```python
from build123d import *

# Parameters (mm, degrees)
SKETCH1_W                   = 88.6
SKETCH1_H                   = 35
BOSS_EXTRUDE1_DEPTH         = 32
TAP_DRILL_FOR_M3X0_5_TAP1_D = 2.5
SKETCH4_W                   = 6.06
SKETCH4_H                   = 35
SKETCH4_W_2                 = 13.02
CUT_EXTRUDE2_DEPTH          = 30
SKETCH5_OUTSIDE_W           = 110.698
SKETCH5_OUTSIDE_H           = 57.098
SKETCH5_OUTSIDE_W_2         = 30
SKETCH5_OUTSIDE_H_2         = 30
CUT_EXTRUDE3_DEPTH          = 10.3
BOSS_EXTRUDE2_DEPTH         = 13.02


with BuildPart() as part:
    # Sketch1 → Boss-Extrude1 (new body)
    with BuildSketch(Plane.XY):
        with Locations((44.3, 17.5)):
            Rectangle(SKETCH1_W, SKETCH1_H)
    extrude(amount=BOSS_EXTRUDE1_DEPTH)

    # Tap Drill for M3x0.5 Tap1 (through all)
    with Locations(Plane.XY.offset(32)):
        with Locations((9.99, 30.535), (9.99, 4.465), (85.57, 4.465), (85.57, 30.535)):
            Hole(TAP_DRILL_FOR_M3X0_5_TAP1_D / 2)

    # Sketch4 → Cut-Extrude2 (cut)
    with BuildSketch(Plane(origin=(0, 0, 0), x_dir=(-1, 0, 0), z_dir=(0, 0, -1))):
        with Locations((-85.57, 17.5)):
            Rectangle(SKETCH4_W, SKETCH4_H)
        with Locations((-6.51, 17.5)):
            Rectangle(SKETCH4_W_2, SKETCH4_H)
    extrude(amount=-CUT_EXTRUDE2_DEPTH, mode=Mode.SUBTRACT)

    # Sketch5 outside → Cut-Extrude3 (cut)
    with BuildSketch(Plane(origin=(0, 0, 0), x_dir=(-1, 0, 0), z_dir=(0, 0, -1))):
        with Locations((-44.3, 17.5)):
            Rectangle(SKETCH5_OUTSIDE_W, SKETCH5_OUTSIDE_H)
        with Locations((-51.54, 17.5)):
            Rectangle(SKETCH5_OUTSIDE_W_2, SKETCH5_OUTSIDE_H_2, mode=Mode.SUBTRACT)
    extrude(amount=-CUT_EXTRUDE3_DEPTH, mode=Mode.SUBTRACT)

    # Sketch6 → Boss-Extrude2 (add)
    with BuildSketch(Plane.ZY.offset(-13.02)):
        with BuildLine():
            Line((19.4, 24.005), (19.4, 10.995))
            ThreePointArc((19.4, 10.995), (14.35, 5.945), (9.3, 10.995))
            Line((9.3, 10.995), (9.3, 24.005))
            ThreePointArc((9.3, 24.005), (14.35, 29.055), (19.4, 24.005))
        make_face()
    extrude(amount=BOSS_EXTRUDE2_DEPTH)


solid = part.part
```
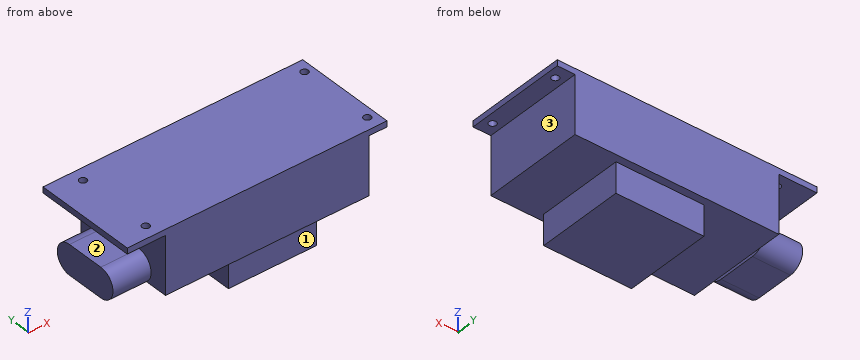
The listing builds one solid part. Answer for the finished solid, in the listing's coordinates (mm). Face numbers are marked on the shaded views. A direction names the side the tool comes from. Round coordinates to 2 decimals unless told otherwise and drop trailing zeros. Loops run counter-clockwise (first coordinate to the right, second up) from the corner with the lowest first, then second, coordinate; pieces in that order, holes last.
Q1. Section D-D, the plane z = 14.35 is taken. Determine the outline of the cut face in (x, y) (3 decimals), then the cut area to 3 significant figures.
Q2. Find the intervals of material crossed by line 1 (Y direction, x = 85.57, z = 30.5) (3 decimals); line 2 (Y direction, x = 85, z = 31); line 3 (X direction, y = 29, z = 10.5), in increasing order.
Q3. Section B-B, the plane y = 12.5 is taken. Determine the outline of the cut face in (x, z).
Q4. Section A-A, the plane x = 85.57 is taken. Determine the outline of the cut face in (y, z) (3 decimals), then the cut area to 3 significant figures.
Q5. Section C-C, the plane x = 9.99 is taken. Determine the outline of the cut face in (y, z) (3 decimals).
Q6. Given pin 1 Ø10 at (y, z) = (17.5, 24) entering from +X; pin 2 Ø8 at (y, z) = (12, 3.5) entering from +X; pin 3 Ø2 at (x, y) = (70.5, 13) entering from -Z, each flat-ended and moving along its own axis, determine where each tip first touches the part or whether it passes through.
Q7. Which of the six approach directions +Z, -Z, +X, -X, +Y, -Y give full straight-line access (tool end or side, diameter ignored) to the marked faces 1, 2 and 3?
Completed:
1. outline: (0, 5.945) - (13.02, 5.945) - (13.02, 0) - (82.54, 0) - (82.54, 35) - (13.02, 35) - (13.02, 29.055) - (0, 29.055) - close
1. area: 2,730 mm2
2. line 1: y = 0 to 3.215, 5.715 to 29.285, 31.785 to 35
2. line 2: y = 0 to 3.35, 5.58 to 29.42, 31.65 to 35
2. line 3: x = 13.02 to 82.54
3. outline: (0, 9.3) - (13.02, 9.3) - (13.02, 10.3) - (36.54, 10.3) - (36.54, 0) - (66.54, 0) - (66.54, 10.3) - (82.54, 10.3) - (82.54, 30) - (88.6, 30) - (88.6, 32) - (0, 32) - (0, 30) - (13.02, 30) - (13.02, 19.4) - (0, 19.4) - close
4. outline: (0, 30) - (3.215, 30) - (3.215, 32) - (0, 32) - close; (5.715, 30) - (29.285, 30) - (29.285, 32) - (5.715, 32) - close; (31.785, 30) - (35, 30) - (35, 32) - (31.785, 32) - close
4. area: 60.0 mm2
5. outline: (0, 30) - (3.215, 30) - (3.215, 32) - (0, 32) - close; (5.715, 30) - (29.285, 30) - (29.285, 32) - (5.715, 32) - close; (10.995, 9.3) - (24.005, 9.3) arc R5.05 ccw to (24.005, 19.4) - (10.995, 19.4) arc R5.05 ccw to start; (31.785, 30) - (35, 30) - (35, 32) - (31.785, 32) - close
6. pin 1: stops at x = 82.54
6. pin 2: stops at x = 66.54
6. pin 3: stops at z = 10.3
7. face 1: -Z, +X, -X, -Y
7. face 2: -X, +Y, -Y
7. face 3: -Z, +X, +Y, -Y
